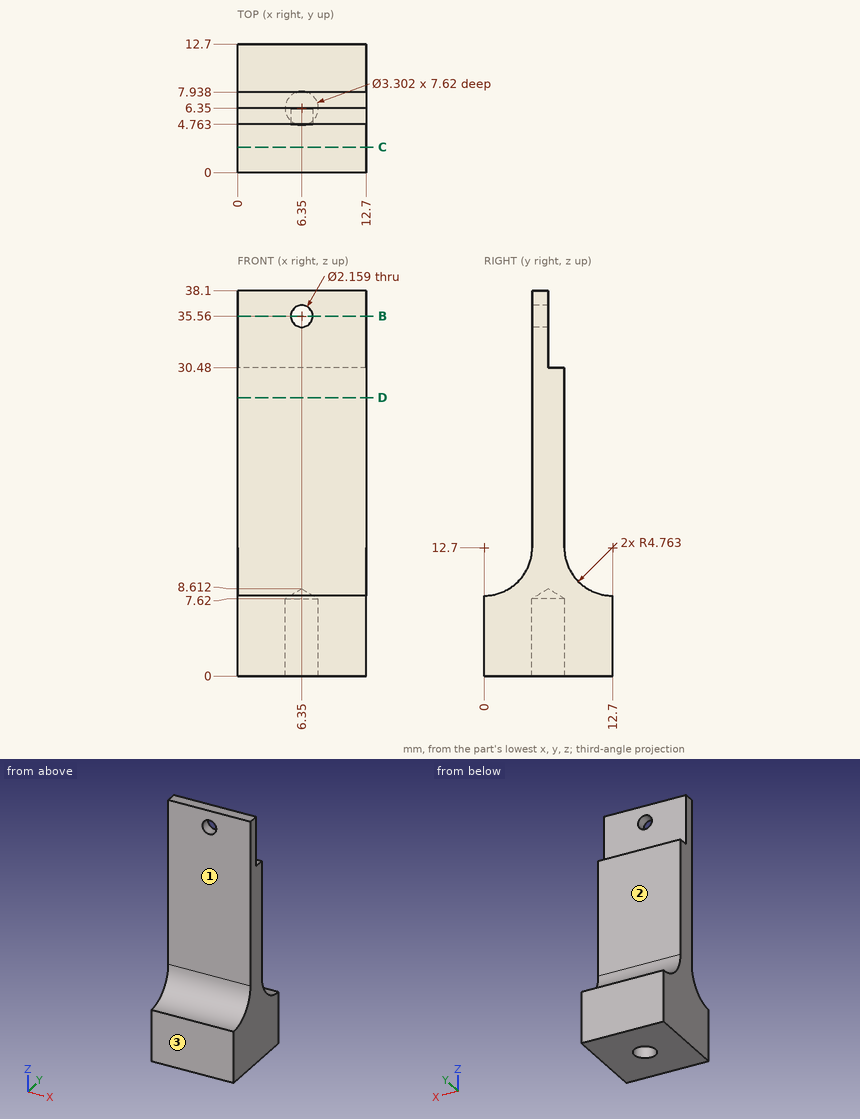
Job drawing, mm, ordinate dimensions from the low corner. One solid piece. A direction names the side the tool comes from. Coordinates: 2 decimals unless noted, no trailing zeros. Order: outer loops, then holes, each group sorted by start corner. A loop starts at its lowest first (then second) coordinate and runs counter-clockwise, first axis right, second up. Notation, with made-up numbers: (-11, 71) -> (16, 71) arc R23 ccw to (16, 104) -> close; hole circle Ø6 at (-0.75, 89). An arc over 180 degrees is marked (long way). Put each result on its own line as item: value. Start each with the question number.
(1) Pin check, flat tips, straight feed: pin 1 Ø3.5 at (x, z) = (6.35, 35.56) entering from -Y; pin 2 Ø4 at (x, z) = (6.5, 35.5) entering from +Y; pin 3 Ø1 at (x, y) = (4.5, 9) entering from -Z; pin 4 Ø4 at (x, z) = (3.5, 13.5) entering from +Y. Stop position of each tip, or through.
(2) Band-saw the part on B-B (z = 35.56). Give the cut face in (x, y).
(3) Band-saw the part on D-D (z = 27.5). Give the cut face in (x, y).
(4) Band-saw the part on C-C (y = 2.5). Give the cut face in (x, z), then the cut area to 3 significant figures.
(5) Which spindle directions (+Z, -Z, +X, -X, +Y, -Y) get a long thin tool onto all of the face, cutting with end or side? Do the marked faces 1, 2 and 3. Say none if no direction does.
(6) Probe line 1 along X through (y, z) = (5.8, 35.56); line 2 along X through (y, z) = (6.35, 5.75). List the from-to ranges inside material, lowest first. Write a range as [from, to].
Determined:
1. pin 1: stops at y = 4.76
1. pin 2: stops at y = 6.35
1. pin 3: stops at z = 0
1. pin 4: stops at y = 8.09
2. outline: (0, 4.76) -> (5.27, 4.76) -> (5.27, 6.35) -> (0, 6.35) -> close; (7.43, 4.76) -> (12.7, 4.76) -> (12.7, 6.35) -> (7.43, 6.35) -> close
3. outline: (0, 4.76) -> (12.7, 4.76) -> (12.7, 7.94) -> (0, 7.94) -> close
4. outline: (0, 0) -> (12.7, 0) -> (12.7, 8.65) -> (0, 8.65) -> close
4. area: 110 mm²
5. face 1: +Z, +X, -X, -Y
5. face 2: +Z, +X, -X, +Y
5. face 3: +Z, -Z, +X, -X, -Y
6. line 1: x = [0, 5.27], [7.43, 12.7]
6. line 2: x = [0, 4.7], [8, 12.7]
